```python
from build123d import *

# Parameters (mm, degrees)
SKETCH_1_R          = 2
EXTRUDE_1_DEPTH     = 2
SKETCH_4_R          = 1.35
SKETCH_4_W          = 8
SKETCH_4_H          = 10
CUT_EXTRUDE_2_DEPTH = 130.341601969
SKETCH_2_R          = 0.75
SKETCH_2_W          = 24
SKETCH_2_H          = 51.5
SKETCH_2_W_2        = 59.5
SKETCH_2_H_2        = 50.064718626
CUT_EXTRUDE_1_DEPTH = 130.341601969
EXTRUDE_1_2_DEPTH   = 2
FILLET_1_R          = 1
FILLET_3_R          = 3
FILLET_2_R          = 2


with BuildPart() as part:
    # 草图1 → Extrude 1 (new body)
    with BuildSketch(Plane(origin=(0, 0, 0), x_dir=(1, 0, 0), z_dir=(0, 1, 0))):
        Polygon((0, 0), (30, 0), (30, 2), (95, 2), (105, -8), (105, -72.5), (83, -72.5), (83, -75.5), (43, -75.5), (43, -72.5), (0, -72.5), align=None)
        with Locations(Location((7.5, -7.5, 0), (0, 0, 270))):
            Circle(SKETCH_1_R, mode=Mode.SUBTRACT)
        with Locations(Location((22.5, -7.5, 0), (0, 0, 270))):
            Circle(SKETCH_1_R, mode=Mode.SUBTRACT)
    extrude(amount=EXTRUDE_1_DEPTH)

    # 草图4 → 切除-拉伸2 (cut, through all)
    with BuildSketch(Plane(origin=(0, 2, 0), x_dir=(1, 0, 0), z_dir=(0, 1, 0))):
        with Locations(Location((34.45, -11.5, 0), (0, 0, 270))):
            Circle(SKETCH_4_R)
        with Locations(Location((46.2, -67.5, 0), (0, 0, 270))):
            Circle(SKETCH_4_R)
        with Locations(Location((90.2, -67.5, 0), (0, 0, 90))):
            Circle(SKETCH_4_R)
        with Locations(Location((101.95, -11.5, 0), (0, 0, 90))):
            Circle(SKETCH_4_R)
        with Locations((68.2, -70.5)):
            Rectangle(SKETCH_4_W, SKETCH_4_H)
    extrude(amount=-CUT_EXTRUDE_2_DEPTH, mode=Mode.SUBTRACT)

    # 草图2 → 切除-拉伸1 (cut, through all)
    with BuildSketch(Plane(origin=(0, 2, 0), x_dir=(1, 0, 0), z_dir=(0, 1, 0))):
        with Locations((83.75, -72.5)):
            Circle(SKETCH_2_R)
        with Locations((42.25, -72.5)):
            Circle(SKETCH_2_R)
        with Locations((18, -40.75)):
            Rectangle(SKETCH_2_W, SKETCH_2_H)
        with Locations((68.2, -34.467640687)):
            Rectangle(SKETCH_2_W_2, SKETCH_2_H_2)
    extrude(amount=-CUT_EXTRUDE_1_DEPTH, mode=Mode.SUBTRACT)

    # 草图3 → Extrude 1 2 (add)
    with BuildSketch(Plane(origin=(0, 2, 0), x_dir=(1, 0, 0), z_dir=(0, 1, 0))):
        Polygon((3.733980422, -16.056009124), (27.733980422, -67.556009124), (32.266019578, -65.443990876), (8.266019578, -13.943990876), align=None)
        Polygon((43.264254449, -7.998436425), (55.764254449, -62.063155051), (60.635745551, -60.936844949), (48.135745551, -6.872126323), align=None)
        Polygon((88.264254449, -6.872126323), (75.764254449, -60.936844949), (80.635745551, -62.063155051), (93.135745551, -7.998436425), align=None)
    extrude(amount=-EXTRUDE_1_2_DEPTH)

    # 圆角1
    fillet_1_edges = [part.edges().sort_by_distance(p)[0] for p in [
        (27.241859665, 1, 66.5),
        (30, 1, 60.581490531),
        (8.758140335, 1, 15),
        (6, 1, 20.918509469),
        (0, 1, 0),
        (30, 1, 0),
        (30, 1, -2),
        (83, 1, 75.5),
        (43, 1, 75.5),
        (0, 1, 72.5),
        (64.2, 1, 65.5),
        (72.2, 1, 65.5),
        (38.45, 1, 59.5),
        (97.95, 1, 59.5),
    ]]
    fillet(fillet_1_edges, radius=FILLET_1_R - 0.0001)  # a hair under: the kernel refuses the full size

    # 圆角3
    fillet_3_edges = [part.edges().sort_by_distance(p)[0] for p in [
        (60.303540699, 1, 59.5),
        (43.596459301, 1, 9.435281374),
        (95, 1, -2),
        (105, 1, 8),
        (92.803540699, 1, 9.435281374),
        (76.096459301, 1, 59.5),
    ]]
    fillet(fillet_3_edges, radius=FILLET_3_R)

    # 圆角2
    fillet_2_edges = [part.edges().sort_by_distance(p)[0] for p in [
        (55.171641763, 1, 59.5),
        (48.728358237, 1, 9.435281374),
        (105, 1, 72.5),
        (81.228358237, 1, 59.5),
        (87.671641763, 1, 9.435281374),
        (6, 1, 66.5),
        (30, 1, 15),
        (38.45, 1, 9.435281374),
        (97.95, 1, 9.435281374),
    ]]
    fillet(fillet_2_edges, radius=FILLET_2_R)


solid = part.part
```
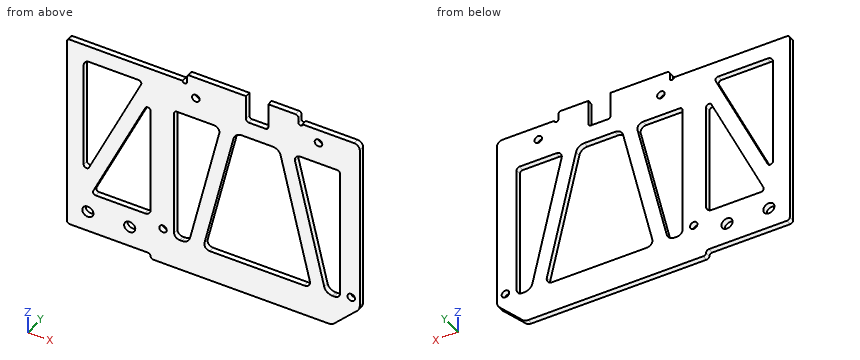
The listing builds one solid part. Answer for the finished solid, in the listing's coordinates (mm). Round coordinates to 2 decimals unless told otherwise and drop trailing zeros. Write each loop counter-clockwise with the first axis right and the second up, starting at its lowest first coordinate (ties: lowest second). Pieces come first, ordered by that corner, then holes. Notation, with made-up numbers: (7.5, 17) -> (50.5, 17) arc R35 ccw to (50.5, 55) -> close; hole circle Ø11 at (87, 45.5). An arc over 180 degrees is marked (long way). Answer as a JSON object with one key per item and string values. Group by question number.
Q1. Section D-D (y = 0.9) is taken. Count the separate pieces of the cut face and the enclosed holes in it, plus the area to 3 significant figures.
Q2. Each of these flat-tipped pins is pushed along its axis until it touches: pin 1 Ø0.6 at (y, z) = (1.5, 74) entering from -X; pin 2 Ø1 at (x, y) = (18.5, 1) entering from -Z; pin 3 Ø0.6 at (x, y) = (17.5, 1) entering from +Z. Where does it stop, or does it pass through?
Q3. Section C-C (x = 22.5) is taken. Write down the section's boundary in (y, z), plus the area to 3 significant figures.
Q4. Straight lines are drawn through the part: line 1 along X through (y, z) = (0.9, 67.5); line 2 along X through (y, z) = (1.9, 31); line 3 along X through (y, z) = (0.4, 7.5). For each, find the intervals that lie inside material, in ascending order.
Q5. Section B-B (z = 51.5) is taken. Write down the section's boundary in (x, y).
Q6. Section A-A (x = 34.45) is taken. Write down the section's boundary in (y, z), plus the area to 3 significant figures.
Check values:
{
 "1": {"separate pieces": "1", "enclosed holes": "11", "area": "4,290 mm^2"},
 "2": {"pin 1": "x = 43", "pin 2": "z = 0", "pin 3": "z = 72.5"},
 "3": {"outline": "(0, 0) -> (2, 0) -> (2, 5.5) -> (0, 5.5) -> close; (0, 9.5) -> (2, 9.5) -> (2, 15) -> (0, 15) -> close; (0, 44.49) -> (2, 44.49) -> (2, 56.32) -> (0, 56.32) -> close; (0, 66.5) -> (2, 66.5) -> (2, 72.5) -> (0, 72.5) -> close", "area": "57.7 mm^2"},
 "4": {"line 1": "0 to 44.85, 47.55 to 64.2, 72.2 to 88.85, 91.55 to 105", "line 2": "0 to 6, 10.7 to 16.21, 30 to 38.45, 48.58 to 53.71, 82.69 to 87.82, 97.95 to 105", "line 3": "0 to 5.5, 9.5 to 20.5, 24.5 to 104.44"},
 "5": {"outline": "(0, 0) -> (6, 0) -> (6, 2) -> (0, 2) -> close; (20.25, 0) -> (25.77, 0) -> (25.77, 2) -> (20.25, 2) -> close; (30, 0) -> (38.45, 0) -> (38.45, 2) -> (30, 2) -> close; (53.32, 0) -> (58.45, 0) -> (58.45, 2) -> (53.32, 2) -> close; (77.95, 0) -> (83.08, 0) -> (83.08, 2) -> (77.95, 2) -> close; (97.95, 0) -> (105, 0) -> (105, 2) -> (97.95, 2) -> close"},
 "6": {"outline": "(0, -2) -> (2, -2) -> (2, 10.15) -> (0, 10.15) -> close; (0, 12.85) -> (2, 12.85) -> (2, 72.5) -> (0, 72.5) -> close", "area": "144 mm^2"}
}
